from build123d import *

# Parameters (mm, degrees)
SKETCH1_W           = 200
SKETCH1_H           = 100
BOSS_EXTRUDE1_DEPTH = 50
SKETCH3_W           = 198.6
SKETCH3_H           = 98.6
CUT_EXTRUDE1_DEPTH  = 49.3
SKETCH4_W           = 54.3
SKETCH4_H           = 98.6
BOSS_EXTRUDE2_DEPTH = 0.7
SKETCH2_R           = 4.5
SKETCH2_R_2         = 1.5
CUT_EXTRUDE2_DEPTH  = 230.128784748
SKETCH8_R           = 1.21
CUT_EXTRUDE6_DEPTH  = 1.8
SKETCH10_R          = 1.87
CUT_EXTRUDE8_DEPTH  = 0.7
SKETCH9_R           = 1.5
CUT_EXTRUDE7_DEPTH  = 213.132034356
SKETCH11_R          = 1.5
CUT_EXTRUDE9_DEPTH  = 0.7


with BuildPart() as part:
    # Sketch1 → Boss-Extrude1 (new body)
    with BuildSketch(Plane(origin=(0, 0, 0), x_dir=(1, 0, 0), z_dir=(0, 1, 0))):
        with Locations((100, 0)):
            Rectangle(SKETCH1_W, SKETCH1_H)
    extrude(amount=BOSS_EXTRUDE1_DEPTH)

    # Sketch3 → Cut-Extrude1 (cut)
    with BuildSketch(Plane.XZ):
        with Locations((100, 0)):
            Rectangle(SKETCH3_W, SKETCH3_H)
    extrude(amount=-CUT_EXTRUDE1_DEPTH, mode=Mode.SUBTRACT)

    # Sketch4 → Boss-Extrude2 (add)
    with BuildSketch(Plane.XZ):
        with Locations((172.15, 0)):
            Rectangle(SKETCH4_W, SKETCH4_H)
    extrude(amount=-BOSS_EXTRUDE2_DEPTH)

    # Sketch2 → Cut-Extrude2 (cut, through all)
    with BuildSketch(Plane.XY.offset(50)):
        with Locations((50, 14)):
            Circle(SKETCH2_R)
        with Locations((50, 4)):
            Circle(SKETCH2_R_2)
        with Locations((50, 24)):
            Circle(SKETCH2_R_2)
    extrude(amount=-CUT_EXTRUDE2_DEPTH, mode=Mode.SUBTRACT)

    # Sketch8 → Cut-Extrude6 (cut)
    with BuildSketch(Plane.XZ):
        with Locations(Location((160, 8.45, 0), (0, 0, 270))):
            Circle(SKETCH8_R)
        with Locations(Location((160, -7.05, 0), (0, 0, 270))):
            Circle(SKETCH8_R)
    extrude(amount=-CUT_EXTRUDE6_DEPTH, mode=Mode.SUBTRACT)

    # Sketch10 → Cut-Extrude8 (cut)
    with BuildSketch(Plane.XZ.offset(-49.3)):
        with Locations(Location((190, 0, 0), (0, 0, 270))):
            Circle(SKETCH10_R)
        with Locations(Location((73, 0, 0), (0, 0, 270))):
            Circle(SKETCH10_R)
    extrude(amount=-CUT_EXTRUDE8_DEPTH, mode=Mode.SUBTRACT)

    # Sketch9 → Cut-Extrude7 (cut, through all)
    with BuildSketch(Plane(origin=(0, 50, 0), x_dir=(1, 0, 0), z_dir=(0, 1, 0))):
        with Locations(Location((15, 0, 0), (0, 0, 270))):
            Circle(SKETCH9_R)
        with Locations(Location((45, 0, 0), (0, 0, 270))):
            Circle(SKETCH9_R)
    extrude(amount=-CUT_EXTRUDE7_DEPTH, mode=Mode.SUBTRACT)

    # Sketch11 → Cut-Extrude9 (cut)
    with BuildSketch(Plane(origin=(143.38, 50, -175.08), x_dir=(0, 0, 1), z_dir=(0, 1, 0))):
        with Locations((129.04, 47)):
            Circle(SKETCH11_R)
        with Locations((181.11, 52.08)):
            Circle(SKETCH11_R)
        with Locations((179.84, 3.82)):
            Circle(SKETCH11_R)
        with Locations((129.04, 19.06)):
            Circle(SKETCH11_R)
    extrude(amount=-CUT_EXTRUDE9_DEPTH, mode=Mode.SUBTRACT)


solid = part.part
CAD build for the part. Positions are in the model's coordinates, mm. A direction names the side the tool comes from. Give positions to 0.01 mm unless a question says otherwise; leave off trailing zeros. Write each loop counter-clockwise with the first axis right and the second up, starting at its lowest first coordinate (ties: lowest second). Pieces come first, ordered by that corner, then holes. Notation, with made-up numbers: M 33.5,46.25 L 86.5,46.25 A9 ccw 86.5,61.25 Z; hole C 66.5,-34.5 d11. An arc over 180 degrees is marked long. Put each result on its own line as item: value. Start each with the question number.
(1) Mould opens along X. For faces 4 (the face through (174, 0, 4)), 5 (the face through (0, 25, 1)), 6 (the face through (99, 24, 49.3)) say: +X half, -X half, draft (parallel to the pull), parting line (faces both ways), or undercut.
(2) Band-saw the part on B-B, the plane z = 17.5. Write the cut outline in (x, y), and give its area (3 significant figures).
(3) Band-saw the part on C-C, the plane y = 33. Write the cut outline in (x, z), and give its area (3 significant figures).
(4) Band-saw the part on A-A, the plane x = 67.5. Write the cut outline in (y, z), and give its area (3 significant figures).
(5) Flat gauge pins, fed straight in: pin 1 Ø3.5 at (x, y) = (50, 4) entering from -Z; pin 2 Ø2.5 at (x, z) = (45, 0) entering from +Y; pin 3 Ø1.8 at (x, z) = (195.46, 6.03) entering from +Y. Where does each tip first touch, or does it go through?
(6) Which spindle directions (+Z, -Z, +X, -X, +Y, -Y) get a long thin tool onto all of the face, cutting with end or side? Do faces 1 (the face through (191.854, 49.645, 0.243)), 2 (the face through (0.7, 24, -1)), 3 (the face through (199.3, 25, -1)). Say none if no direction does.
(7) Probe L1, parallel to Y at x = 50, z = 49.45; L2, parallel to X at y = 49.7, z = 0; L3, parallel to Z at x = 73, y = 49. List the from-to ranges inside material, lowest first.
Response values:
1. face 4: draft
1. face 5: -X half
1. face 6: undercut
2. outline: M 0,0 L 0.7,0 L 0.7,49.3 L 199.3,49.3 L 199.3,0.7 L 145,0.7 L 145,0 L 200,0 L 200,50 L 0,50 Z
2. area: 247 mm2
3. outline: M 0,-50 L 200,-50 L 200,50 L 0,50 Z; hole M 0.7,-49.3 L 199.3,-49.3 L 199.3,49.3 L 0.7,49.3 Z
3. area: 418 mm2
4. outline: M 0,-50 L 50,-50 L 50,50 L 0,50 L 0,49.3 L 49.3,49.3 L 49.3,-49.3 L 0,-49.3 Z
4. area: 139 mm2
5. pin 1: stops at z = -50
5. pin 2: passes through
5. pin 3: stops at y = 0.7
6. face 1: +Y
6. face 2: -Y
6. face 3: none
7. L1: y = 0 to 2.5, 5.5 to 9.5, 18.5 to 22.5, 25.5 to 50
7. L2: x = 0 to 13.5, 16.5 to 43.5, 46.5 to 71.13, 74.87 to 188.13, 191.87 to 200
7. L3: z = -50 to -49.3, 49.3 to 50
